Can you work these out from the drawing? Everything is in mm from the part's minimum corner. A direction names the side the tool comes from. Round coordinates to 2 decimals unless told otherwise and drop trailing zeros. Loops run counter-clockwise (first coordinate to the right, second up) from the corner with the lowest first, then second, coordinate; pieces in that order, holes last. Notation, with made-up numbers: (28, -31.5) -> (46, -31.5) arc R7 ccw to (46, -25.5) -> close; hole circle Ø3 at (3.25, 64.25). An arc over 180 degrees is marked (long way). One line per item, written item: value.
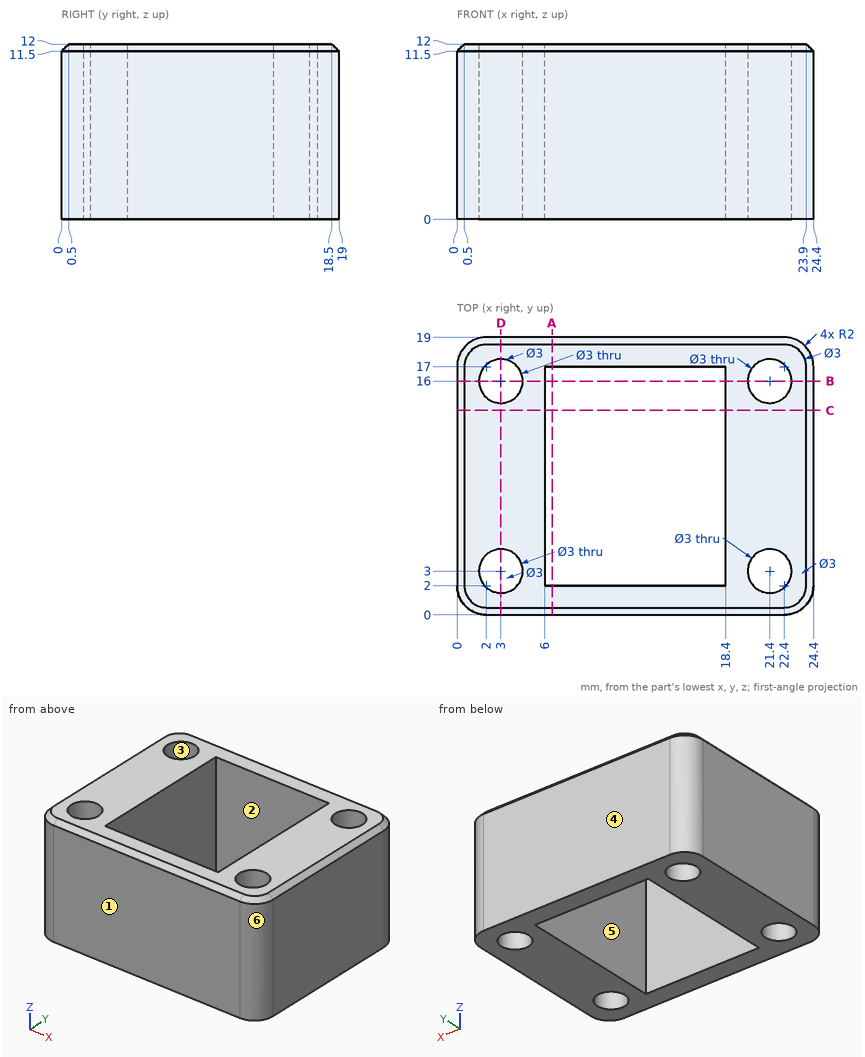
Item 1: If we section it at D-D on x = 3: List the corners of the cut face in (y, z) for me, plus the area to 3 significant figures.
Output:
outline: (0, 0) -> (1.5, 0) -> (1.5, 12) -> (0.5, 12) -> (0, 11.5) -> close; (4.5, 0) -> (14.5, 0) -> (14.5, 12) -> (4.5, 12) -> close; (17.5, 0) -> (19, 0) -> (19, 11.5) -> (18.5, 12) -> (17.5, 12) -> close
area: 156 mm²
Item 2: Will these pins go through, and if not, where does the flat tip stop? pin 1 Ø3.5 at (x, y) = (3, 16) entering from +Z; pin 2 Ø1.8 at (x, y) = (3, 3) entering from +Z.
Output:
pin 1: stops at z = 12
pin 2: passes through
Item 3: If we mould it in two halves opening along X, with no side actions, what happens to the marked faces 3, 4, 5 and 6? For each: released by +X, released by -X, zero draft, split by the parting line, or undercut.
Output:
face 3: undercut
face 4: zero draft
face 5: undercut
face 6: released by +X
Item 4: I need wall thicknesses on line 1 (Y direction, x = 21.4, z = 6.75); line 2 (X direction, y = 12, z = 3.5); line 3 (Y direction, x = 6.5, z = 3.5). Which ranges of each line are inside material? Lowest first, please. Write a range as from..to.
Output:
line 1: y = 0..1.5, 4.5..14.5, 17.5..19
line 2: x = 0..6, 18.4..24.4
line 3: y = 0..2, 17..19
Item 5: If we section it at A-A on x = 6.5: List the corners of the cut face in (y, z) for me, plus the area to 4 significant figures.
Output:
outline: (0, 0) -> (2, 0) -> (2, 12) -> (0.5, 12) -> (0, 11.5) -> close; (17, 0) -> (19, 0) -> (19, 11.5) -> (18.5, 12) -> (17, 12) -> close
area: 47.75 mm²
Item 6: If we section it at B-B on y = 16: List the corners of the cut face in (x, z) for me, plus the area to 4 significant figures.
Output:
outline: (0, 0) -> (1.5, 0) -> (1.5, 12) -> (0.5, 12) -> (0, 11.5) -> close; (4.5, 0) -> (6, 0) -> (6, 12) -> (4.5, 12) -> close; (18.4, 0) -> (19.9, 0) -> (19.9, 12) -> (18.4, 12) -> close; (22.9, 0) -> (24.4, 0) -> (24.4, 11.5) -> (23.9, 12) -> (22.9, 12) -> close
area: 71.75 mm²
Item 7: If we section it at C-C on y = 14: List the corners of the cut face in (x, z) for me, plus the area to 3 significant figures.
Output:
outline: (0, 0) -> (6, 0) -> (6, 12) -> (0.5, 12) -> (0, 11.5) -> close; (18.4, 0) -> (24.4, 0) -> (24.4, 11.5) -> (23.9, 12) -> (18.4, 12) -> close
area: 144 mm²
Item 8: For the marked faces 1 and 2, which set-ups out of +Z, -Z, +X, -X, +Y, -Y let a thin tool reach every point of the face, with its end or its side?
Output:
face 1: +Z, -Z, +X, -X, -Y
face 2: +Z, -Z
